Autodesk Inventor part; units mm, degrees
ref_plane "YZ Plane" through (0, 0, 0) normal (1, 0, 0) x (0, 1, 0)
ref_plane "XZ Plane" through (0, 0, 0) normal (0, 1, 0) x (-1, 0, 0)
ref_plane "XY Plane" through (0, 0, 0) normal (0, 0, 1) x (1, 0, 0)
sketch "Sketch1" plane through (0, 0, 0) normal (0, 1, 0) x (-1, 0, 0)
  line L0 (-12.7, 25.4) -> (12.7, 25.4)
  line L1 (12.7, 25.4) -> (12.7, -12.7)
  line L2 (12.7, -12.7) -> (-12.7, -12.7)
  line L3 (-12.7, -12.7) -> (-12.7, 25.4)
  line L4 (-12.7, 0) -> (12.7, 0) construction
  circle A0 centre (0, 12.7) radius 6.35
  circle A1 centre (9.525, 22.225) radius 1.5875
  circle A2 centre (-9.525, 3.175) radius 1.5875
  circle A3 centre (-7.9375, -6.35) radius 2.1526
  circle A4 centre (7.9375, -6.35) radius 2.1526
  point P0 (0, 0)
  point P1 (0, 0)
  dimension "d0" = 12.7
  dimension "d2" = 25.4
  dimension "d3" = 25.4
  dimension "d4" = 12.7
  dimension "d5" = 3.175
  dimension "d6" = 3.175
  dimension "d7" = 4.3053
  dimension "d8" = 4.3053
  dimension "d9" = 3.175
  dimension "d10" = 3.175
  dimension "d11" = 3.175
  dimension "d12" = 3.175
  dimension "d13" = 12.7
  dimension "d14" = 12.7
  dimension "d15" = 6.35
  dimension "d16" = 6.35
  dimension "d17" = 15.875
  dimension "d18" = 4.7625
extrude "Extrusion1" add sketch "Sketch1" along normal blind 0.7874
equation "\"d15\" = 0.5 * d0"
equation "\"d16\" = d15"
equation "\"d18\" = -0.5 * d17 + 0.5 * d2"
properties part number "launcher_hinge"
Here's how the part is built. I have some questions about the finished solid (model axes, mm). Round coordinates to 2 decimals unless told otherwise and drop trailing zeros. Loops run counter-clockwise (first coordinate to the right, second up) from the corner with the lowest first, then second, coordinate; pieces in that order, holes last.
1. Suppose I cut it at A-A, the plane z = -6.35. Please give me the cut outline in (x, y).
Answers:
outline: (-12.7, 0) - (-10.09, 0) - (-10.09, 0.79) - (-12.7, 0.79) - close; (-5.78, 0) - (5.78, 0) - (5.78, 0.79) - (-5.78, 0.79) - close; (10.09, 0) - (12.7, 0) - (12.7, 0.79) - (10.09, 0.79) - close
2. Suppose I cut it at C-C, the plane z = 12.7. Please give me the cut outline in (x, y), and give its area (4 significant figures).
Answers:
outline: (-12.7, 0) - (-6.35, 0) - (-6.35, 0.79) - (-12.7, 0.79) - close; (6.35, 0) - (12.7, 0) - (12.7, 0.79) - (6.35, 0.79) - close
area: 10.00 mm2
3. Will this pin go through, and if not, where does the flat tip stop? pin 1 (2.5 mm diameter, centred on x = 9.525, z = 3.175, fed in from -Y).
Answers:
pin 1: passes through
4. Thinking about a two-plate mould opening in Z: for faces 1 (the face through (1.38, 0.39, 18.9)), 2 (the face through (-2.6, 0, 6.6)), which applies, released by +Z, released by -Z, zero draft, split by the parting line, or undercut?
Answers:
face 1: undercut
face 2: zero draft
5. If I drill on probe 1 along Z at (x, y) = (0, 0.5); probe 2 along Z at (x, y) = (-9.25, 0.3); probe 3 along Z at (x, y) = (9.75, 0.25), over which ranges is the centre line in solid material (lowest first)?
Answers:
probe 1: z = -12.7 to 6.35, 19.05 to 25.4
probe 2: z = -12.7 to -8.06, -4.64 to 20.66, 23.79 to 25.4
probe 3: z = -12.7 to -7.51, -5.19 to 1.6, 4.75 to 25.4
6. Suppose I cut it at B-B, the plane x = 0. Please give me the cut outline in (y, z).
Answers:
outline: (0, -12.7) - (0.79, -12.7) - (0.79, 6.35) - (0, 6.35) - close; (0, 19.05) - (0.79, 19.05) - (0.79, 25.4) - (0, 25.4) - close
7. Suppose I cut it at D-D, the plane y = 0.4. Give the number of separate pieces and of enclosed holes in the cut face, and give its area (3 significant figures).
Answers:
separate pieces: 1
enclosed holes: 5
area: 796 mm2
